Answer from the drawing. Dimensions are ordinates in mm from the lowest x, y and z of the part. Give positions to 0.01 mm unless a question says otherwise; leave off trailing zeros. Order: outer loops, then holes, each group sorted by start corner. A loop starts at its lowest first (then second) coordinate and runs counter-clockwise, first axis right, second up.
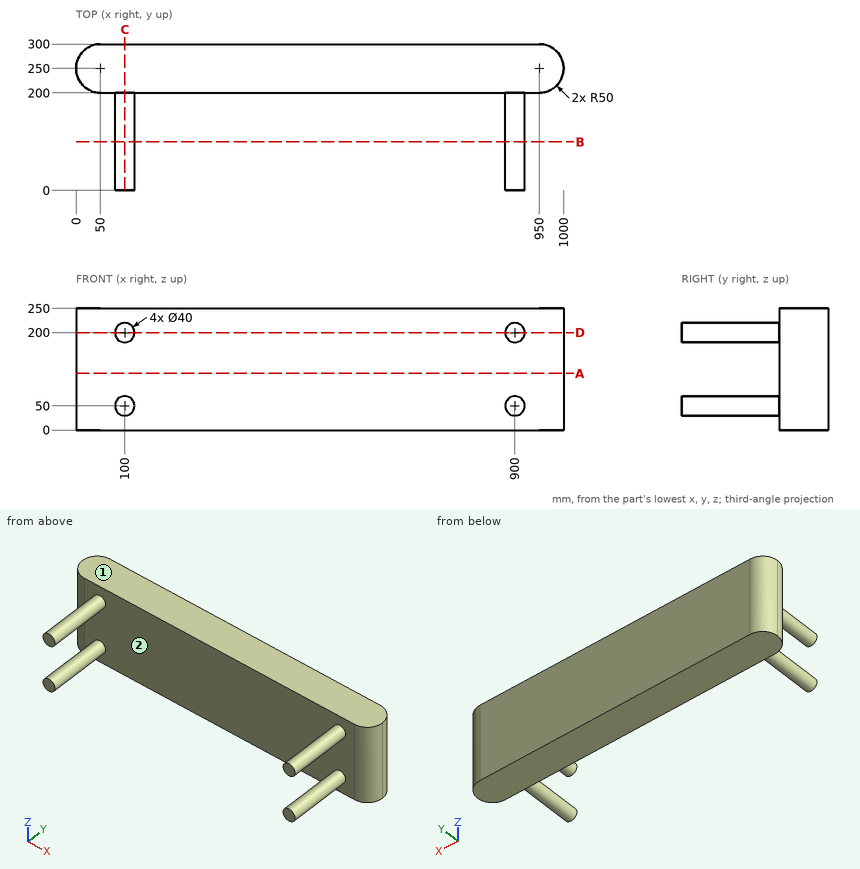
1) The part is cut by section B-B on y = 99.5. Determine the outline of the cut face in (x, z).
Final values:
outline: circle Ø40 at (100, 50); circle Ø40 at (100, 200); circle Ø40 at (900, 50); circle Ø40 at (900, 200)
2) The part is cut by section C-C on x = 100. Determine the outline of the cut face in (y, z), and give its area (3 significant figures).
Final values:
outline: (0, 30) - (200, 30) - (200, 0) - (300, 0) - (300, 250) - (200, 250) - (200, 220) - (0, 220) - (0, 180) - (200, 180) - (200, 70) - (0, 70) - close
area: 41,000 mm2
3) The part is cut by section D-D on z = 200. Determine the outline of the cut face in (x, y).
Final values:
outline: (50, 200) - (80, 200) - (80, 0) - (120, 0) - (120, 200) - (880, 200) - (880, 0) - (920, 0) - (920, 200) - (950, 200) arc R50 ccw to (950, 300) - (50, 300) arc R50 ccw to start
4) Given pin 1 (2 mm diameter, centred on y = 109, z = 63.5, fed in from +X); pin 2 (4 mm diameter, centred on y = 209.5, z = 134.5, fed in from +X); pin 3 (10 mm diameter, centred on y = 99, z = 203, fed in from +X), each flat-ended and moving along its own axis, determine where each tip first touches the part or whether it passes through.
Final values:
pin 1: stops at x = 915.61
pin 2: stops at x = 981.9
pin 3: stops at x = 920
5) For a pull along X with two mould halves and no side action, classify the marked faces 1 and 2 as released by +X, released by -X, zero draft, split by the parting line, or undercut.
Final values:
face 1: zero draft
face 2: undercut
6) Consider L1, parallel to Y at x = 116.5, z = 227; L2, parallel to X at y = 149, z = 50; L3, parallel to X at y = 232.5, z = 204.5. Determine where each line is inside the solid, lowest interval first.
Final values:
L1: y = 200 to 300
L2: x = 80 to 120, 880 to 920
L3: x = 3.16 to 996.84
7) The part is cut by section A-A on z = 116.5. Determine the outline of the cut face in (x, y).
Final values:
outline: (50, 200) - (950, 200) arc R50 ccw to (950, 300) - (50, 300) arc R50 ccw to start
